from build123d import *

# Parameters (mm, degrees)
SKETCH1_W                       = 100
SKETCH1_H                       = 100
BOSS_EXTRUDE1_DEPTH             = 95
SKETCH2_W                       = 10
SKETCH2_H                       = 10
BOSS_EXTRUDE2_DEPTH             = 105
SKETCH3_R                       = 1.4
CUT_EXTRUDE1_DEPTH              = 10
SKETCH4_W                       = 11
SKETCH4_H                       = 11
BOSS_EXTRUDE3_DEPTH             = 105
SKETCH5_R                       = 1.4
CUT_EXTRUDE2_DEPTH              = 10
SKETCH6_R                       = 1.4
CUT_EXTRUDE3_DEPTH              = 10
CHAMFER1_SIZE                   = 1
SKETCH7_W                       = 19
SKETCH7_H                       = 43
SKETCH7_W_2                     = 16
SKETCH7_H_2                     = 40
BOSS_EXTRUDE4_DEPTH             = 3
SKETCH8_W                       = 16
SKETCH8_H                       = 40
CUT_EXTRUDE4_DEPTH              = 10
CHAMFER2_SIZE                   = 13
SKETCH9_W                       = 16
SKETCH9_H                       = 3.1
CUT_EXTRUDE5_DEPTH              = 10
FILLET1_R                       = 1
SKETCH10_R                      = 1.4
CUT_EXTRUDE6_DEPTH              = 10
SKETCH11_R                      = 5
BOSS_EXTRUDE5_DEPTH             = 3
SKETCH12_W                      = 30.5
SKETCH12_H                      = 2.2
CUT_EXTRUDE7_DEPTH              = 3
SKETCH13_W                      = 30.5
SKETCH13_H                      = 2.2
CUT_EXTRUDE8_DEPTH              = 3
SKETCH14_W                      = 2.2
SKETCH14_H                      = 30.5
CUT_EXTRUDE9_DEPTH              = 3
CUT_EXTRUDE10_DEPTH             = 45
CUT_EXTRUDE10_DEPTH_BACK        = 45
SKETCH15_W                      = 90
SKETCH15_H                      = 58
CUT_EXTRUDE11_REACH             = 125.296
CUT_EXTRUDE11_DIRECTION_2_REACH = 125.296
CHAMFER3_SIZE                   = 4
SKETCH17_W                      = 102
SKETCH17_H                      = 53.035118915
CUT_EXTRUDE12_DEPTH             = 152.673992497
SKETCH19_W                      = 95
SKETCH19_H                      = 95
CUT_EXTRUDE14_DEPTH             = 12
SKETCH20_R                      = 1.6
CUT_EXTRUDE15_DEPTH             = 152.003311222
SKETCH21_R                      = 1.6
CUT_EXTRUDE16_DEPTH             = 152.003311222


with BuildPart() as part:
    # Sketch1 → Boss-Extrude1 (new body)
    with BuildSketch(Plane(origin=(0, 0, 0), x_dir=(1, 0, 0), z_dir=(0, 1, 0))):
        Rectangle(SKETCH1_W, SKETCH1_H)
    extrude(amount=BOSS_EXTRUDE1_DEPTH)

    # Sketch2 → Boss-Extrude2 (add)
    with BuildSketch(Plane(origin=(0, 100, 0), x_dir=(1, 0, 0), z_dir=(0, 1, 0))):
        with Locations((-45, 45)):
            Rectangle(SKETCH2_W, SKETCH2_H)
        with Locations((45, 45)):
            Rectangle(SKETCH2_W, SKETCH2_H)
        with Locations((45, -45)):
            Rectangle(SKETCH2_W, SKETCH2_H)
        with Locations((-45, -45)):
            Rectangle(SKETCH2_W, SKETCH2_H)
    extrude(amount=-BOSS_EXTRUDE2_DEPTH)

    # Sketch3 → Cut-Extrude1 (cut)
    with BuildSketch(Plane(origin=(0, 95, 0), x_dir=(1, 0, 0), z_dir=(0, 1, 0))):
        with Locations(Location((-28, -45, 0), (0, 0, 270))):
            Circle(SKETCH3_R)
        with Locations(Location((28, -45, 0), (0, 0, 90))):
            Circle(SKETCH3_R)
        with Locations(Location((28, 45, 0), (0, 0, 270))):
            Circle(SKETCH3_R)
        with Locations(Location((-28, 45, 0), (0, 0, 90))):
            Circle(SKETCH3_R)
    cut_extrude1 = extrude(amount=-CUT_EXTRUDE1_DEPTH, mode=Mode.SUBTRACT)

    # Sketch4 → Boss-Extrude3 (add)
    with BuildSketch(Plane(origin=(0, 100, 0), x_dir=(1, 0, 0), z_dir=(0, 1, 0))):
        with Locations((-45.5, 45.5)):
            Rectangle(SKETCH4_W, SKETCH4_H)
        with Locations((45.5, 45.5)):
            Rectangle(SKETCH4_W, SKETCH4_H)
        with Locations((45.5, -45.5)):
            Rectangle(SKETCH4_W, SKETCH4_H)
        with Locations((-45.5, -45.5)):
            Rectangle(SKETCH4_W, SKETCH4_H)
    extrude(amount=-BOSS_EXTRUDE3_DEPTH)

    # Sketch5 → Cut-Extrude2 (cut)
    with BuildSketch(Plane.XY.offset(50)):
        with Locations((-36, 91)):
            Circle(SKETCH5_R)
        with Locations(Location((36, 91, 0), (0, 0, 180))):
            Circle(SKETCH5_R)
        with Locations((36, 4)):
            Circle(SKETCH5_R)
        with Locations(Location((-36, 4, 0), (0, 0, 180))):
            Circle(SKETCH5_R)
    cut_extrude2 = extrude(amount=-CUT_EXTRUDE2_DEPTH, mode=Mode.SUBTRACT)

    # Mirror1: Cut-Extrude2 across plane
    add(cut_extrude2.mirror(Plane.XY), mode=Mode.SUBTRACT)

    # Sketch6 → Cut-Extrude3 (cut)
    with BuildSketch(Plane.ZY.offset(50)):
        with Locations((-36, 91)):
            Circle(SKETCH6_R)
        with Locations(Location((36, 91, 0), (0, 0, 180))):
            Circle(SKETCH6_R)
        with Locations((36, 4)):
            Circle(SKETCH6_R)
        with Locations(Location((-36, 4, 0), (0, 0, 180))):
            Circle(SKETCH6_R)
    cut_extrude3 = extrude(amount=-CUT_EXTRUDE3_DEPTH, mode=Mode.SUBTRACT)

    # Mirror2: Cut-Extrude3 across plane
    add(cut_extrude3.mirror(Plane(origin=(0, 0, 0), x_dir=(0, 0, 1), z_dir=(1, 0, 0))), mode=Mode.SUBTRACT)

    # Mirror3: Cut-Extrude1 across plane
    add(cut_extrude1.mirror(Plane.ZX.offset(47.5)), mode=Mode.SUBTRACT)

    # Chamfer1
    chamfer1_edges = [part.edges().sort_by_distance(p)[0] for p in [
        (-45.5, -5, 51),
        (-51, -5, 45.5),
        (-51, 100, 45.5),
        (-45.5, 100, 51),
        (51, -5, 45.5),
        (45.5, -5, 51),
        (45.5, 100, 51),
        (51, 100, 45.5),
        (45.5, -5, -51),
        (51, -5, -45.5),
        (51, 100, -45.5),
        (45.5, 100, -51),
        (-51, -5, -45.5),
        (-45.5, -5, -51),
        (-45.5, 100, -51),
        (-51, 100, -45.5),
        (-45.5, -5, 40),
        (-40, -5, 45.5),
        (-40, 100, 45.5),
        (-45.5, 100, 40),
        (40, -5, 45.5),
        (45.5, -5, 40),
        (45.5, 100, 40),
        (40, 100, 45.5),
        (45.5, -5, -40),
        (40, -5, -45.5),
        (45, 95, -40),
        (40, 100, -45.5),
        (45.5, 100, -40),
        (-40, -5, -45.5),
        (-45.5, -5, -40),
        (-45.5, 100, -40),
        (-40, 100, -45.5),
    ]]
    chamfer(chamfer1_edges, length=CHAMFER1_SIZE)

    # Sketch7 → Boss-Extrude4 (add)
    with BuildSketch(Plane(origin=(0, 95, 0), x_dir=(1, 0, 0), z_dir=(0, 1, 0))):
        with Locations((0, -17)):
            Rectangle(SKETCH7_W, SKETCH7_H)
        with Locations((0, -17)):
            Rectangle(SKETCH7_W_2, SKETCH7_H_2, mode=Mode.SUBTRACT)
    extrude(amount=BOSS_EXTRUDE4_DEPTH)

    # Sketch8 → Cut-Extrude4 (cut)
    with BuildSketch(Plane(origin=(0, 95, 0), x_dir=(1, 0, 0), z_dir=(0, 1, 0))):
        with Locations((0, -17)):
            Rectangle(SKETCH8_W, SKETCH8_H)
    extrude(amount=-CUT_EXTRUDE4_DEPTH, mode=Mode.SUBTRACT)

    # Chamfer2
    chamfer2_edges = [part.edges().sort_by_distance(p)[0] for p in [
        (0, 85, 37),
    ]]
    chamfer(chamfer2_edges, length=CHAMFER2_SIZE - 0.0001)  # a hair under: the kernel refuses the full size

    # Sketch9 → Cut-Extrude5 (cut)
    with BuildSketch(Plane(origin=(0, 85, 0), x_dir=(1, 0, 0), z_dir=(0, 1, 0))):
        with Locations((0, 1.45)):
            Rectangle(SKETCH9_W, SKETCH9_H)
    extrude(amount=-CUT_EXTRUDE5_DEPTH, mode=Mode.SUBTRACT)

    # Fillet1
    fillet1_edges = [part.edges().sort_by_distance(p)[0] for p in [
        (0, 85, 0.1),
    ]]
    fillet(fillet1_edges, radius=FILLET1_R)

    # Sketch10 → Cut-Extrude6 (cut)
    with BuildSketch(Plane.XY.offset(-3)):
        with Locations((0, 92)):
            Circle(SKETCH10_R)
    extrude(amount=-CUT_EXTRUDE6_DEPTH, mode=Mode.SUBTRACT)

    # Sketch11 → Boss-Extrude5 (add)
    with BuildSketch(Plane.XZ):
        with Locations(Location((0, -15, 0), (0, 0, 90))):
            Circle(SKETCH11_R)
    extrude(amount=BOSS_EXTRUDE5_DEPTH)

    # Sketch12 → Cut-Extrude7 (cut)
    with BuildSketch(Plane.ZY.offset(50)):
        with Locations((0, 74.4)):
            Rectangle(SKETCH12_W, SKETCH12_H)
        with Locations((0, 20.6)):
            Rectangle(SKETCH12_W, SKETCH12_H)
    cut_extrude7 = extrude(amount=-CUT_EXTRUDE7_DEPTH, mode=Mode.SUBTRACT)

    # Mirror4: Cut-Extrude7 across plane
    add(cut_extrude7.mirror(Plane(origin=(0, 0, 0), x_dir=(0, 0, 1), z_dir=(1, 0, 0))), mode=Mode.SUBTRACT)

    # Sketch13 → Cut-Extrude8 (cut)
    with BuildSketch(Plane.XY.offset(50)):
        with Locations((0, 74.4)):
            Rectangle(SKETCH13_W, SKETCH13_H)
        with Locations((0, 20.6)):
            Rectangle(SKETCH13_W, SKETCH13_H)
    cut_extrude8 = extrude(amount=-CUT_EXTRUDE8_DEPTH, mode=Mode.SUBTRACT)

    # Mirror5: Cut-Extrude8 across plane
    add(cut_extrude8.mirror(Plane.XY), mode=Mode.SUBTRACT)

    # Sketch14 → Cut-Extrude9 (cut)
    with BuildSketch(Plane(origin=(0, 95, 0), x_dir=(1, 0, 0), z_dir=(0, 1, 0))):
        with Locations((26.9, 0)):
            Rectangle(SKETCH14_W, SKETCH14_H)
        with Locations((-26.9, 0)):
            Rectangle(SKETCH14_W, SKETCH14_H)
    cut_extrude9 = extrude(amount=-CUT_EXTRUDE9_DEPTH, mode=Mode.SUBTRACT)

    # Mirror6: Cut-Extrude9 across plane
    add(cut_extrude9.mirror(Plane.ZX.offset(47.5)), mode=Mode.SUBTRACT)

    # Sketch15 → Cut-Extrude10 (cut, two sides: drawn at the far end of the back side and taken through both)
    with BuildSketch(Plane(origin=(0, 0, 0), x_dir=(0, 0, -1), z_dir=(1, 0, 0)).offset(-CUT_EXTRUDE10_DEPTH_BACK)):
        with Locations((0, 41)):
            Rectangle(SKETCH15_W, SKETCH15_H)
    extrude(amount=CUT_EXTRUDE10_DEPTH + CUT_EXTRUDE10_DEPTH_BACK, mode=Mode.SUBTRACT)

    # Cut-Extrude11: up to this face of the body (flat: up to its plane)
    cut_extrude11_end = Plane(part.part.faces().sort_by_distance((0, 41, 45))[0])
    # Sketch16 → Cut-Extrude11 (cut, up to the picked face)
    with BuildSketch(Plane.XY, mode=Mode.PRIVATE) as cut_extrude11_sk1:
        Polygon((45, 57.006357685), (-45, 57.006357685), (-45, 83), (-13, 83), (-13, 67.006357685), (13, 67.006357685), (13, 83), (45, 83), align=None)
    cut_extrude11_tool1 = split(extrude(cut_extrude11_sk1.sketch, amount=CUT_EXTRUDE11_REACH, mode=Mode.PRIVATE), bisect_by=cut_extrude11_end, keep=Keep.BOTH, mode=Mode.PRIVATE)
    add(cut_extrude11_tool1.solids().sort_by(Axis((0, 57.943143, 0), (0, 0, 1)))[0], mode=Mode.SUBTRACT)

    # Cut-Extrude11 direction 2: up to this face of the body (flat: up to its plane)
    cut_extrude11_direction_2_end = Plane(part.part.faces().sort_by_distance((0, 41, -45))[0])
    # Sketch16 → Cut-Extrude11 direction 2 (cut, up to the picked face)
    with BuildSketch(Plane.XY, mode=Mode.PRIVATE) as cut_extrude11_direction_2_sk1:
        Polygon((45, 57.006357685), (-45, 57.006357685), (-45, 83), (-13, 83), (-13, 67.006357685), (13, 67.006357685), (13, 83), (45, 83), align=None)
    cut_extrude11_direction_2_tool1 = split(extrude(cut_extrude11_direction_2_sk1.sketch, amount=-CUT_EXTRUDE11_DIRECTION_2_REACH, mode=Mode.PRIVATE), bisect_by=cut_extrude11_direction_2_end, keep=Keep.BOTH, mode=Mode.PRIVATE)
    add(cut_extrude11_direction_2_tool1.solids().sort_by(Axis((0, 57.943143, 0), (0, 0, -1)))[0], mode=Mode.SUBTRACT)

    # Chamfer3
    chamfer3_edges = [part.edges().sort_by_distance(p)[0] for p in [
        (13, 70, 0),
        (-13, 70, 0),
    ]]
    chamfer(chamfer3_edges, length=CHAMFER3_SIZE)

    # Sketch17 → Cut-Extrude12 (cut, through all)
    with BuildSketch(Plane(origin=(51, 0, 0), x_dir=(0, 0, -1), z_dir=(1, 0, 0))):
        with Locations((0, 15.982440543)):
            Rectangle(SKETCH17_W, SKETCH17_H)
    extrude(amount=-CUT_EXTRUDE12_DEPTH, mode=Mode.SUBTRACT)

    # Sketch19 → Cut-Extrude14 (cut)
    with BuildSketch(Plane.XZ.offset(-42.5)):
        Rectangle(SKETCH19_W, SKETCH19_H)
    extrude(amount=-CUT_EXTRUDE14_DEPTH, mode=Mode.SUBTRACT)

    # Sketch20 → Cut-Extrude15 (cut, through all)
    with BuildSketch(Plane(origin=(50, 0, 0), x_dir=(0, 0, -1), z_dir=(1, 0, 0))):
        with Locations((0, 47.5)):
            Circle(SKETCH20_R)
    extrude(amount=-CUT_EXTRUDE15_DEPTH, mode=Mode.SUBTRACT)

    # Sketch21 → Cut-Extrude16 (cut, through all)
    with BuildSketch(Plane(origin=(0, 0, -50), x_dir=(-1, 0, 0), z_dir=(0, 0, -1))):
        with Locations((0, 47.5)):
            Circle(SKETCH21_R)
    extrude(amount=-CUT_EXTRUDE16_DEPTH, mode=Mode.SUBTRACT)


solid = part.part
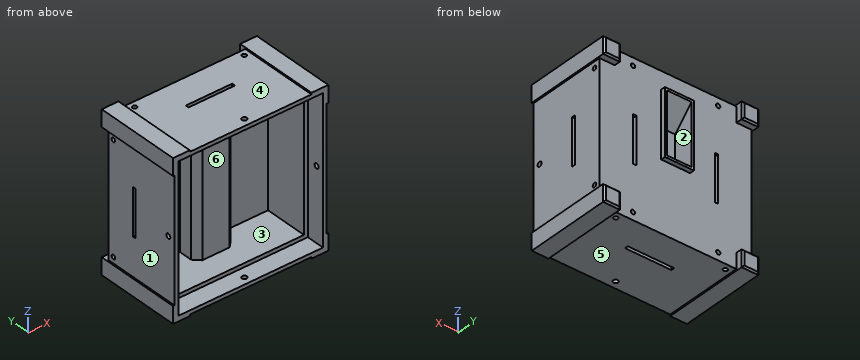
Geometry: final body of the model. Coordinates: model frame, mm. Face numbers are marked on the shaded views. A direction names the side the tool comes from. Give positions to 0.01 mm unless a question says otherwise; leave off trailing zeros. Order: outer loops, then holes, each group sorted by start corner. A loop starts at its lowest first (then second) coordinate and runs counter-clockwise, first axis right, second up. Notation, with made-up numbers: (0.5, 88) -> (21.5, 88) arc R29 cw to (21.5, 119) -> close; hole circle Ø7 at (-6, 20). An arc over 180 degrees is marked (long way). Write each question's results on one line, items separated by ' | '.
1) Cut plane B-B (x = -43). Output: boundary loops of the cut face in (y, z).
Geometry says:
outline: (42.5, -51) -> (99, -51) -> (100, -50) -> (100, -41) -> (99, -40) -> (95, -40) -> (95, 40) -> (99, 40) -> (100, 41) -> (100, 50) -> (99, 51) -> (42.5, 51) -> (42.5, 47.5) -> (54.5, 47.5) -> (54.5, 45) -> (83, 45) -> (83, -45) -> (54.5, -45) -> (54.5, -47.5) -> (42.5, -47.5) -> close; hole circle Ø2.8 at (91, -36); hole circle Ø2.8 at (91, 36)
2) First-contact query: pin 1 Ø2 at (y, z) = (48.5, -1.5) entering from -X; pin 2 Ø3 at (x, z) = (-28, 45) entering from +Y; pin 3 Ø1.1 at (x, y) = (27, 93.5) entering from +Z; pin 4 Ø12 at (x, y) = (-36, 71) entering from -Z. Flat tips, straight axial feed; report the tip coordinate or a pass-through.
Geometry says:
pin 1: stops at x = -50 | pin 2: stops at y = 95 | pin 3: stops at z = 50 | pin 4: stops at z = -51
3) Line query: line 1 along X through (y, z) = (89, -45); line 2 along Z through (x, y) = (26.5, 81). Output: solid intervals per line, ascending.
Geometry says:
line 1: x = -51 to -29.4, -26.6 to 26.6, 29.4 to 51 | line 2: z = -50 to -45, 45 to 50
4) Cut plane C-C (x = 0). Give the number of separate pieces and of enclosed holes in the cut face, and give its area (3 significant figures).
Geometry says:
separate pieces: 3 | enclosed holes: 0 | area: 2,320 mm²
5) Draft query along Z for the marked faces 4, 5 and 6. Return one class per face: released by +Z, released by -Z, zero draft, split by the parting line, or undercut.
Geometry says:
face 4: released by +Z | face 5: released by -Z | face 6: undercut
6) Set-up query: the marked faces 1, 2 and 3. Return all of +Z, -Z, +X, -X, +Y, -Y with unobstructed straight access to the full face (end or side cutting, diameter ignored); none if empty.
Geometry says:
face 1: -X, +Y, -Y | face 2: +Y | face 3: -Y
7) Cut plane A-A (y = 60). Output: boundary loops of the cut face in (x, z).
Geometry says:
outline: (-51, -51) -> (-40, -51) -> (-40, -50) -> (40, -50) -> (40, -51) -> (51, -51) -> (51, -40) -> (50, -40) -> (50, 40) -> (51, 40) -> (51, 51) -> (40, 51) -> (40, 50) -> (-40, 50) -> (-40, 51) -> (-51, 51) -> (-51, 40) -> (-50, 40) -> (-50, -40) -> (-51, -40) -> close; hole (-45, -45) -> (45, -45) -> (45, 45) -> (-45, 45) -> close
